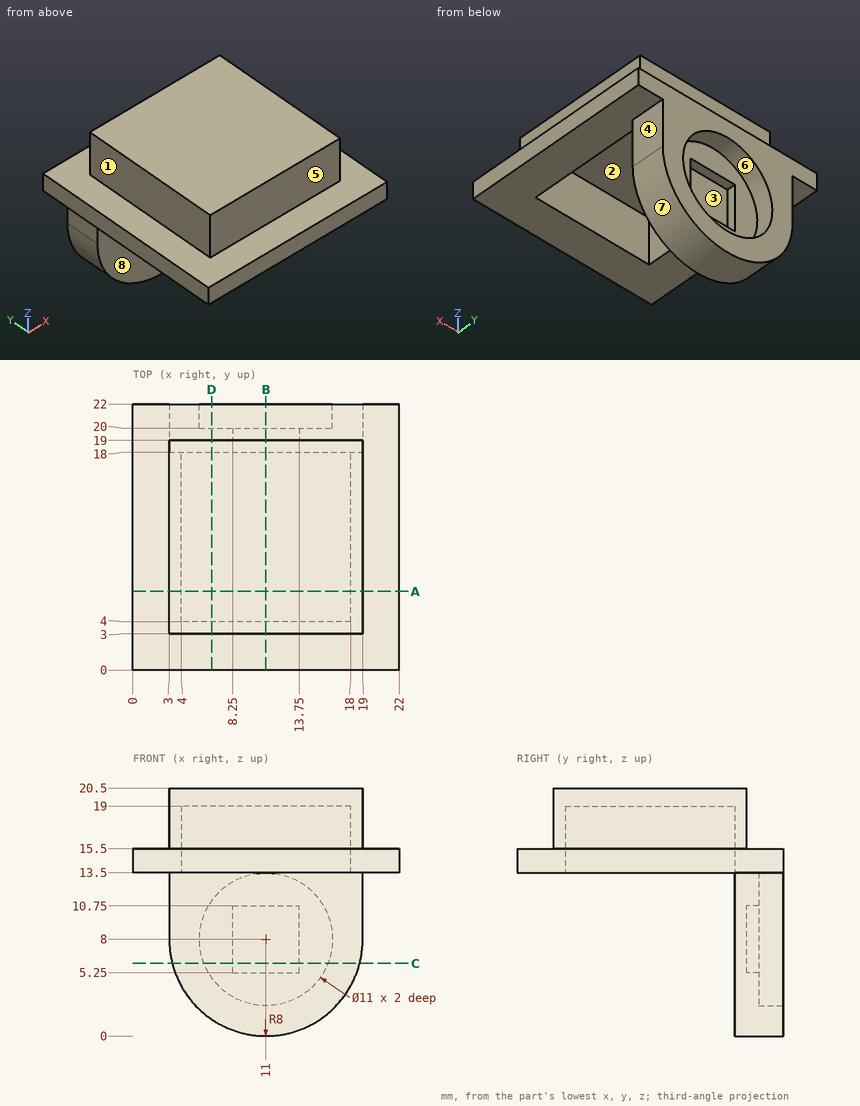
Geometry: see drawing. Coordinates: mm, zero at the bounding-box minimum. A direction names the side the tool comes from. Coordinates: 2 decimals unless noted, no trailing zeros. Order: outer loops, then holes, each group sorted by start corner. A loop starts at its lowest first (then second) coordinate and runs counter-clockwise, first axis right, second up. Notation, with made-up numbers: (-12.5, 62.5) - (6.5, 62.5) arc R22 cw to (6.5, 94.5) - close; hole circle Ø2 at (76.5, 1). An arc over 180 degrees is marked (long way). Write each question's results on one line, items separated by ' | '.
1) Section A-A, the plane y = 6.5. Return loops of the section in (x, z).
Results list:
outline: (0, 13.5) - (4, 13.5) - (4, 19) - (18, 19) - (18, 13.5) - (22, 13.5) - (22, 15.5) - (19, 15.5) - (19, 20.5) - (3, 20.5) - (3, 15.5) - (0, 15.5) - close
2) Set-up query: the marked faces 1, 2, 3, 4 and 5. Return all of +Z, -Z, +X, -X, +Y, -Y with unobstructed straight access to the full face (end or side cutting, diameter ignored); none if empty.
Results list:
face 1: +Z, -X, +Y, -Y | face 2: -Z | face 3: +Y | face 4: -Z, +X, +Y, -Y | face 5: +Z, +X, -X, -Y
3) Section B-B, the plane x = 11. Return loops of the section in (y, z), plus the area to 3 significant figures.
Results list:
outline: (0, 13.5) - (4, 13.5) - (4, 19) - (18, 19) - (18, 0) - (22, 0) - (22, 2.5) - (20, 2.5) - (20, 5.25) - (19, 5.25) - (19, 10.75) - (20, 10.75) - (20, 13.5) - (22, 13.5) - (22, 15.5) - (19, 15.5) - (19, 20.5) - (3, 20.5) - (3, 15.5) - (0, 15.5) - close | area: 73.5 mm^2
4) Section D-D, the plane x = 6.5. Return loops of the section in (y, z).
Results list:
outline: (0, 13.5) - (4, 13.5) - (4, 19) - (18, 19) - (18, 1.39) - (22, 1.39) - (22, 4.84) - (20, 4.84) - (20, 11.16) - (22, 11.16) - (22, 15.5) - (19, 15.5) - (19, 20.5) - (3, 20.5) - (3, 15.5) - (0, 15.5) - close
5) Section C-C, the plane z = 6. Return loops of the section in (x, y), plus the area to 3 significant figures.
Results list:
outline: (3.25, 18) - (18.75, 18) - (18.75, 22) - (16.12, 22) - (16.12, 20) - (13.75, 20) - (13.75, 19) - (8.25, 19) - (8.25, 20) - (5.88, 20) - (5.88, 22) - (3.25, 22) - close | area: 36.0 mm^2
6) Pin query (flat end, axial travel): pin 1 (3.5 mm diameter, centred on x = 13, z = 7, fed in from +Y); pin 2 (8 mm diameter, centred on x = 5.5, y = 7.5, fed in from -Z); pin 3 (4 mm diameter, centred on y = 15, z = 14.5, fed in from -X); pin 4 (1.6 mm diameter, centred on y = 13, z = 16.5, fed in from +X). Return the tip coordinate at first contact, or that it passes through.
Results list:
pin 1: y = 20 | pin 2: z = 13.5 | pin 3: x = 0 | pin 4: x = 19
7) Line query: line 1 (Z direction, x = 11, y = 20.4); line 2 (X direction, y = 6.25, z = 18); line 3 (Z direction, x = 3.75, y = 11.5). Output: solid intervals per line, ascending. Write a range as from..to.
Results list:
line 1: 0..2.5, 13.5..15.5 | line 2: 3..4, 18..19 | line 3: 13.5..20.5
8) Pull-direction query (Z, two-part tool) for the marked faces 6, 7 and 8; classes: pulls with the +Z half, pulls with the -Z half, needs draft (parallel to the pull), parting line crosses it, or undercut.
Results list:
face 6: undercut | face 7: pulls with the -Z half | face 8: needs draft
